The listing builds one solid part. Answer for the finished solid, in the listing's coordinates (mm). Round coordinates to 2 decimals unless told otherwise and drop trailing zeros. Write each loop counter-clockwise with the first axis right and the second up, starting at its lowest first coordinate (ties: lowest second). Pieces come first, ordered by that corner, then holes. Notation, with made-up numbers: (-22.5, 33.25) - (17.5, 33.25) arc R11 ccw to (17.5, 43.25) - close; hole circle Ø2 at (59, -22.5). An arc over 180 degrees is marked (long way). Use a Markdown table: item, result. Add a question column.
1) Each of these flat-tipped pins is pushed along its axis until it touches: P1, Ø5.5, axis at x = 0, z = -41.275, coming from the -Y side; P2, Ø1, axis at y = 1.5, z = 32, coming from the -X side. Where does it stop, or does it pass through?
2) A cutting plane is placed at D-D (y = 1.1). State how many separate pieces and enclosed holes the cut face has, then the cut area to 3 significant figures.
3) A cutting plane is placed at B-B (x = -13.5). Give the vertices of the cut face in (y, z), then the cut area to 3 significant figures.
4) A cutting plane is placed at A-A (x = 0). Give the vertices of the cut face in (y, z) (3 decimals), then the cut area to 3 significant figures.
5) A cutting plane is placed at C-C (z = 20). Give the vertices of the cut face in (x, y).
6) Find the intervals of material crossed by probe 1 along Z at (x, y) = (-34.5, 1.2); probe 2 along X at (y, z) = (1, 20); probe 3 along Z at (x, y) = (36, 0.6), in increasing order. Write a range as from..to.
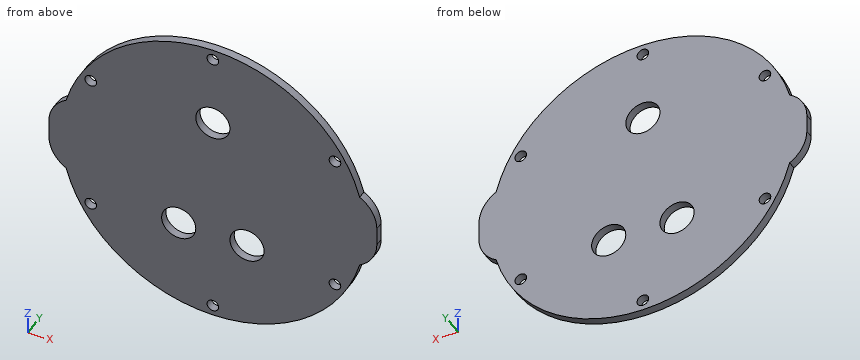
```python
from build123d import *

# Parameters (mm, degrees)
BOSS_EXTRUDE1_DEPTH  = 2.4
M3_CLEARANCE_HOLE1_D = 3.4
CIRPATTERN1_COUNT    = 6
SKETCH8_R            = 5
CUT_EXTRUDE2_DEPTH   = 66.464207778


with BuildPart() as part:
    # Sketch1 → Boss-Extrude1 (new body)
    with BuildSketch(Plane(origin=(0, 0, 0), x_dir=(1, 0, 0), z_dir=(0, 1, 0))):
        with BuildLine():
            ThreePointArc((-42.969094344, -11.378024049), (-44.45, 0), (-42.969094344, 11.378024049))
            ThreePointArc((-42.969094344, 11.378024049), (-46.651327743, 7.715429023), (-48, 2.7))
            Line((-48, 2.7), (-48, -2.7))
            ThreePointArc((-48, -2.7), (-46.651327743, -7.715429023), (-42.969094344, -11.378024049))
        make_face()
        with BuildLine():
            Line((38, 12.7), (-38, 12.7))
            ThreePointArc((-38, 12.7), (-40.570968641, 12.363856386), (-42.969094344, 11.378024049))
            ThreePointArc((-42.969094344, 11.378024049), (-44.45, 0), (-42.969094344, -11.378024049))
            ThreePointArc((-42.969094344, -11.378024049), (-40.570968641, -12.363856386), (-38, -12.7))
            Line((-38, -12.7), (38, -12.7))
            ThreePointArc((38, -12.7), (40.570968641, -12.363856386), (42.969094344, -11.378024049))
            ThreePointArc((42.969094344, -11.378024049), (44.078218791, -5.736996445), (44.45, 0))
            ThreePointArc((44.45, 0), (44.078218791, 5.736996445), (42.969094344, 11.378024049))
            ThreePointArc((42.969094344, 11.378024049), (40.570968641, 12.363856386), (38, 12.7))
        make_face()
        with BuildLine():
            ThreePointArc((-38, -12.7), (-40.570968641, -12.363856386), (-42.969094344, -11.378024049))
            ThreePointArc((-42.969094344, -11.378024049), (0, -44.45), (42.969094344, -11.378024049))
            ThreePointArc((42.969094344, -11.378024049), (40.570968641, -12.363856386), (38, -12.7))
            Line((38, -12.7), (-38, -12.7))
        make_face()
        with BuildLine():
            ThreePointArc((-42.969094344, 11.378024049), (-40.570968641, 12.363856386), (-38, 12.7))
            Line((-38, 12.7), (38, 12.7))
            ThreePointArc((38, 12.7), (40.570968641, 12.363856386), (42.969094344, 11.378024049))
            ThreePointArc((42.969094344, 11.378024049), (0, 44.45), (-42.969094344, 11.378024049))
        make_face()
        with BuildLine():
            ThreePointArc((48, 2.7), (46.651327743, 7.715429023), (42.969094344, 11.378024049))
            ThreePointArc((42.969094344, 11.378024049), (44.078218791, 5.736996445), (44.45, 0))
            ThreePointArc((44.45, 0), (44.078218791, -5.736996445), (42.969094344, -11.378024049))
            ThreePointArc((42.969094344, -11.378024049), (46.651327743, -7.715429023), (48, -2.7))
            Line((48, -2.7), (48, 2.7))
        make_face()
    extrude(amount=BOSS_EXTRUDE1_DEPTH)

    # M3 Clearance Hole1 (through all)
    with Locations(Plane(origin=(0, 2.4, -41.275), x_dir=(0, 0, 1), z_dir=(0, 1, 0))):
        with Locations((0, 0)):
            m3_clearance_hole1 = Hole(M3_CLEARANCE_HOLE1_D / 2)

    # CirPattern1: M3 Clearance Hole1 ×6 about axis
    cirpattern1_axis = Axis((0, 0, 0), (0, 1, 0))
    for i in range(1, CIRPATTERN1_COUNT):
        add(m3_clearance_hole1.rotate(cirpattern1_axis, i * 360 / CIRPATTERN1_COUNT), mode=Mode.SUBTRACT)

    # Sketch8 → Cut-Extrude2 (cut, through all)
    with BuildSketch(Plane(origin=(0, 2.4, 0), x_dir=(1, 0, 0), z_dir=(0, 1, 0))):
        with Locations(Location((-10, 17.320508076, 0), (0, 0, 270))):
            Circle(SKETCH8_R)
        with Locations(Location((10, 17.320508076, 0), (0, 0, 90))):
            Circle(SKETCH8_R)
        with Locations(Location((0, -20, 0), (0, 0, 270))):
            Circle(SKETCH8_R)
    extrude(amount=-CUT_EXTRUDE2_DEPTH, mode=Mode.SUBTRACT)


solid = part.part
```
Entries:
| question | item | result |
|---|---|---|
| 1 | P1 | stops at y = 0 |
| 1 | P2 | stops at x = -31.36 |
| 2 | separate pieces | 1 |
| 2 | enclosed holes | 9 |
| 2 | area | 6,050 mm² |
| 3 | outline | (0, -42.35) - (2.4, -42.35) - (2.4, -20.89) - (0, -20.89) - close; (0, -13.75) - (2.4, -13.75) - (2.4, 42.35) - (0, 42.35) - close |
| 3 | area | 186 mm² |
| 4 | outline | (0, -44.45) - (2.4, -44.45) - (2.4, -42.975) - (0, -42.975) - close; (0, -39.575) - (2.4, -39.575) - (2.4, 15) - (0, 15) - close; (0, 25) - (2.4, 25) - (2.4, 39.575) - (0, 39.575) - close; (0, 42.975) - (2.4, 42.975) - (2.4, 44.45) - (0, 44.45) - close |
| 4 | area | 173 mm² |
| 5 | outline | (-39.7, 0) - (-37.32, 0) - (-37.32, 2.4) - (-39.7, 2.4) - close; (-34.17, 0) - (-5, 0) - (-5, 2.4) - (-34.17, 2.4) - close; (5, 0) - (34.17, 0) - (34.17, 2.4) - (5, 2.4) - close; (37.32, 0) - (39.7, 0) - (39.7, 2.4) - (37.32, 2.4) - close |
| 6 | probe 1 | z = -28.03..-21.79, -19.48..19.48, 21.79..28.03 |
| 6 | probe 2 | x = -39.7..-37.32, -34.17..-5, 5..34.17, 37.32..39.7 |
| 6 | probe 3 | z = -26.07..-22.32, -18.96..18.96, 22.32..26.07 |
